Check sheet for the modelled part. Datum: model origin and axes. Units: mm. Face numbers are marked on the shaded views. A direction names the side the tool comes from. Coordinates: 2 decimals unless noted, no trailing zeros. Loops run counter-clockwise (first coordinate to the right, second up) from the corner with the lowest first, then second, coordinate; pieces in that order, holes last. Notation, with made-up numbers: M 20.25,72 L 57.25,72 A32 cw 57.25,100 Z; hole C -22,-17 d9. An arc over 180 degrees is marked long. Write each question's results on one line, items separated by ' | '. Start each with the question number.
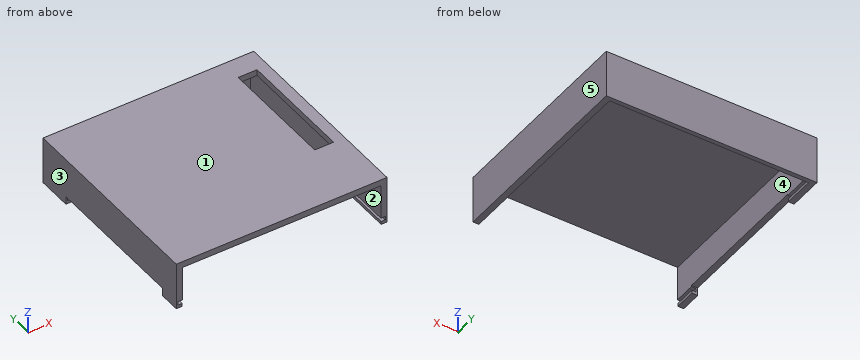
from build123d import *

# Parameters (mm, degrees)
BOSS_EXTRUDE1_DEPTH      = 1
BOSS_EXTRUDE1_DEPTH_BACK = 95
SKETCH3_W                = 102.168296719
SKETCH3_H                = 23.073037812
BOSS_EXTRUDE2_DEPTH      = 2
CUT_EXTRUDE1_DEPTH       = 7
SKETCH5_W                = 9.153790551
SKETCH5_H                = 56.288421304
CUT_EXTRUDE2_DEPTH       = 12


with BuildPart() as part:
    # Sketch1 → Boss-Extrude1 (new, two sides: drawn at the far end of the back side and taken through both)
    with BuildSketch(Plane(origin=(1.86e-07, 2.18892535, 0), x_dir=(0.9999999999999963, -8.499370700000005e-08, 0), z_dir=(-8.499370700000005e-08, -0.9999999999999964, 0)).offset(-BOSS_EXTRUDE1_DEPTH_BACK)):
        Polygon((-10.086587255, 78.390258261), (-12.920734899, 78.390258261), (-12.920734899, 101.463296073), (89.24756182, 101.463296073), (89.24756182, 78.390258261), (86.413414176, 78.390258261), (86.413414176, 79.890257832), (88.421490182, 79.890257832), (88.421490182, 81.69025819), (86.24756182, 81.69025819), (86.24756182, 98.463296073), (-9.920734899, 98.463296073), (-9.920734899, 81.69025819), (-12.094663261, 81.69025819), (-12.094663261, 79.890257832), (-10.086587255, 79.890257832), align=None)
    extrude(amount=BOSS_EXTRUDE1_DEPTH + BOSS_EXTRUDE1_DEPTH_BACK)

    # Sketch3 → Boss-Extrude2 (add)
    with BuildSketch(Plane(origin=(8.26e-06, 97.18892535, 0), x_dir=(0.9999999999999963, -8.499370702344177e-08, 0), z_dir=(8.499370702344177e-08, 0.9999999999999964, 0))):
        with Locations((38.163413461, -89.926777167)):
            Rectangle(SKETCH3_W, SKETCH3_H)
    extrude(amount=BOSS_EXTRUDE2_DEPTH)

    # Sketch4 → Cut-Extrude1 (cut)
    with BuildSketch(Plane(origin=(-12.920734899, 1.098e-06, 0), x_dir=(0, 0, 1), z_dir=(-0.9999999999999964, 8.499370700000005e-08, 0))):
        Polygon((78.390258261, 11.48892535), (82.313500316, 11.48892535), (82.313500316, 82.388929164), (78.390258261, 82.388929164), (75.766454091, 82.388929164), (75.766454091, 11.48892535), align=None)
    extrude(amount=-CUT_EXTRUDE1_DEPTH, mode=Mode.SUBTRACT)

    # Sketch5 → Cut-Extrude2 (cut)
    with BuildSketch(Plane.XY.offset(101.463296073)):
        with Locations((79.217116041, 60.318884388)):
            Rectangle(SKETCH5_W, SKETCH5_H)
    extrude(amount=-CUT_EXTRUDE2_DEPTH, mode=Mode.SUBTRACT)


solid = part.part
Item 1: Depth check by flat-ended pin: P1, Ø5, axis at x = 39.5, y = 72, coming from the -Z side; P2, Ø1.2, axis at y = 62.5, z = 79, coming from the -X side; P3, Ø10, axis at x = 40, z = 83.5, coming from the -Y side. Enter the tip coordinate at first touch or a pass-through.
Item 2: Section check A-A (x = 77). Record the cut outline in (y, z), plus the area to 3 significant figures.
Item 3: Release check for a two-part mould opening along X. For the marked faces 3, 4 and 5 record: +X half, -X half, draft (parallel to the pull), parting line (faces both ways), or undercut.
Item 4: Section check B-B (y = 41). Record the cut outline in (x, z), plus the area to 3 significant figures.
Item 5: Tool access check on the marked faces 1 and 2. Record the directions out of +Z, -Z, +X, -X, +Y, -Y that give a thin tool (end or side, any length) a straight path to the whole face; none if there is none.
Item 6: Section check D-D (y = 10). Record the cut outline in (x, z).
Item 7: Thickness scan on line 1 (X direction, y = 21.5, z = 86.75); line 2 (Y direction, x = 48, z = 85); line 3 (Z direction, x = 83, y = 23). Record the ranges inside material, lowest first.
Item 8: Section check C-C (z = 87.75). Record the cut outline in (x, y).
Computed values:
1) P1: stops at z = 98.46 | P2: stops at x = 86.41 | P3: stops at y = 97.19
2) outline: M 1.19,98.46 L 32.17,98.46 L 32.17,101.46 L 1.19,101.46 Z; M 88.46,98.46 L 97.19,98.46 L 97.19,78.39 L 99.19,78.39 L 99.19,101.46 L 88.46,101.46 Z | area: 165 mm²
3) face 3: -X half | face 4: undercut | face 5: +X half
4) outline: M -12.92,82.31 L -9.92,82.31 L -9.92,98.46 L 74.64,98.46 L 74.64,101.46 L -12.92,101.46 Z; M 83.79,98.46 L 86.25,98.46 L 86.25,81.69 L 88.42,81.69 L 88.42,79.89 L 86.41,79.89 L 86.41,78.39 L 89.25,78.39 L 89.25,101.46 L 83.79,101.46 Z | area: 384 mm²
5) face 1: +Z, +X, -X, +Y, -Y | face 2: -Z, -Y
6) outline: M -12.92,78.39 L -10.09,78.39 L -10.09,79.89 L -12.09,79.89 L -12.09,81.69 L -9.92,81.69 L -9.92,98.46 L 86.25,98.46 L 86.25,81.69 L 88.42,81.69 L 88.42,79.89 L 86.41,79.89 L 86.41,78.39 L 89.25,78.39 L 89.25,101.46 L -12.92,101.46 Z
7) line 1: x = -12.92 to -9.92, 86.25 to 89.25 | line 2: y = 97.19 to 99.19 | line 3: z = 98.46 to 101.46
8) outline: M -12.92,1.19 L -9.92,1.19 L -9.92,97.19 L 86.25,97.19 L 86.25,1.19 L 89.25,1.19 L 89.25,99.19 L -12.92,99.19 Z
